For this review, take the finished solid that the model builds, in its own axes (mm). A direction names the side the tool comes from. Coordinates: 2 decimals unless noted, no trailing zeros. Write each loop counter-clockwise with the first axis right and the second up, starting at its lowest first coordinate (ties: lowest second). Pieces come first, ordered by that corner, then holes. Notation, with made-up numbers: M -22,44.25 L 8,44.25 A23 ccw 8,73.25 Z; hole C 43.5,61.25 d9. An arc over 180 degrees is marked long. One line per question, with ' | ' between items.
from build123d import *

# Parameters (mm, degrees)
SKETCH1_W           = 39.05
SKETCH1_H           = 76.2
BOSS_EXTRUDE1_DEPTH = 3
SKETCH2_W           = 3
SKETCH2_H           = 15
CUT_EXTRUDE1_DEPTH  = 73.446802019
LPATTERN1_COUNT     = 3
LPATTERN1_PITCH     = 22.8


with BuildPart() as part:
    # Sketch1 → Boss-Extrude1 (new body)
    with BuildSketch(Plane.XY):
        with Locations((-21.468460648, -21.557986111)):
            Rectangle(SKETCH1_W, SKETCH1_H)
    extrude(amount=BOSS_EXTRUDE1_DEPTH)

    # Sketch2 → Cut-Extrude1 (cut, through all)
    with BuildSketch(Plane.XY.offset(3)):
        with Locations((-39.493460648, 1.242013889)):
            Rectangle(SKETCH2_W, SKETCH2_H)
        with Locations((-3.443460648, 1.242013889)):
            Rectangle(SKETCH2_W, SKETCH2_H)
    cut_extrude1 = extrude(amount=-CUT_EXTRUDE1_DEPTH, mode=Mode.SUBTRACT)

    # LPattern1: Cut-Extrude1 ×3
    with Locations(*[(0, -i * LPATTERN1_PITCH, 0) for i in range(1, LPATTERN1_COUNT)]):
        add(cut_extrude1, mode=Mode.SUBTRACT)


solid = part.part
1) We need section B-B on y = 2.5. State the section outline as (x, z) points.
Responses:
outline: M -37.99,0 L -4.94,0 L -4.94,3 L -37.99,3 Z
2) Insertion check: pin 1 Ø1.5 at (y, z) = (-22, 1) entering from -X; pin 2 Ø10 at (x, y) = (-22, -15.5) entering from -Z. Each pin has a flat end and moves straight along its axis. Give the tip position at first contact, or say it passes through.
Responses:
pin 1: x = -37.99 | pin 2: z = 0
3) We need section A-A on z = 2.35. State the section outline as (x, y) points, then the cut area to 3 significant figures.
Responses:
outline: M -40.99,-59.66 L -1.94,-59.66 L -1.94,-51.86 L -4.94,-51.86 L -4.94,-36.86 L -1.94,-36.86 L -1.94,-29.06 L -4.94,-29.06 L -4.94,-14.06 L -1.94,-14.06 L -1.94,-6.26 L -4.94,-6.26 L -4.94,8.74 L -1.94,8.74 L -1.94,16.54 L -40.99,16.54 L -40.99,8.74 L -37.99,8.74 L -37.99,-6.26 L -40.99,-6.26 L -40.99,-14.06 L -37.99,-14.06 L -37.99,-29.06 L -40.99,-29.06 L -40.99,-36.86 L -37.99,-36.86 L -37.99,-51.86 L -40.99,-51.86 Z | area: 2,710 mm^2
4) Machinability: for faces 1 (the flat face through (-40, 8.742, 2)), 2 (the flat face through (-3, -29.058, 2)), 3 (the flat face through (-22, -21, 3)), which of the approach directions +Z, -Z, +X, -X, +Y, -Y give a long, thin tool a straight path to every point of the face, cutting with its end or side? Answer none if there is none.
Responses:
face 1: +Z, -Z, -X | face 2: +Z, -Z, +X | face 3: +Z, +X, -X, +Y, -Y
5) The part is to be moulded in two halves that separate along Y. For faces 4 (the flat face through (-40, -36.858, 2)), 5 (the flat face through (-4.943, 1, 2)), 6 (the flat face through (-40.993, -56, 1)), 7 (the flat face through (-22, 16.542, 1)), say which applies: +Y half, -Y half, draft (parallel to the pull), parting line (faces both ways), or undercut.
Responses:
face 4: undercut | face 5: undercut | face 6: draft | face 7: +Y half
6) To check wall thickness, follow line 1 along X through (y, z) = (-39.5, 1.15). State the ranges of the line that lie inside material, in increasing order. Write a range as [from, to].
Responses:
line 1: [-37.99, -4.94]
